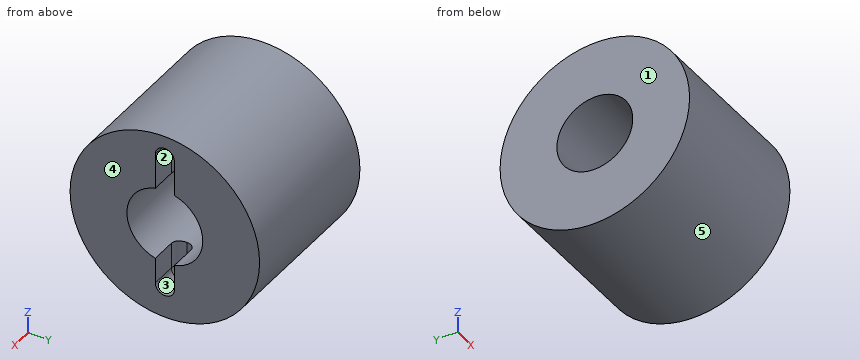
```python
from build123d import *

# Parameters (mm, degrees)
F0_R     = 14.985
F0_R_2   = 6
F1_DEPTH = 25
F3_DEPTH = 5.5
F4_R     = 1.5


with BuildPart() as f1:
    # F0 (on Right) → F1 (new body)
    with BuildSketch(Plane.YZ):
        Circle(F0_R)
        Circle(F0_R_2, mode=Mode.SUBTRACT)
    extrude(amount=-F1_DEPTH)

    # F2 (on Right) → F3 (cut)
    with BuildSketch(Plane.YZ):
        with BuildLine():
            ThreePointArc((1.51, 11.49), (0, 13), (-1.51, 11.49))
            Line((-1.51, 11.49), (-1.51, -9.89))
            ThreePointArc((-1.51, -9.89), (0, -11.4), (1.51, -9.89))
            Line((1.51, -9.89), (1.51, 11.49))
        make_face()
    extrude(amount=-F3_DEPTH, mode=Mode.SUBTRACT)

    # F4
    f4_edges = [f1.edges().sort_by_distance(p)[0] for p in [
        (-5.5, 1.51, 8.648442),
        (-5.5, 1.51, -7.848442),
    ]]
    fillet(f4_edges, radius=F4_R)


solid = f1.part
```
Work out the finished part from the listing and answer in its coordinate system (mm). Face numbers are marked on the shaded views. A direction names the side the tool comes from. Give positions to 0.01 mm unless a question says otherwise; leave off trailing zeros. Write each loop counter-clockwise with the first axis right and the second up, starting at its lowest first coordinate (ties: lowest second). Pieces come first, ordered by that corner, then holes. Notation, with made-up numbers: (-30.75, 30) -> (-1.75, 30) arc R21 cw to (-1.75, 66) -> close; hole circle Ø7 at (-30, 81). An arc over 180 degrees is marked (long way). Write item = value, one per line.
Q1. Consider line 1 along Z through (x, y) = (-18, 0) (3 decimals); line 2 along Y through (x, z) = (-13, 1); line 3 along Y through (x, z) = (-4.25, 11). Determine where each line is inside the solid, lowest interval first.
Computed values:
line_1 = -14.985 to -6, 6 to 14.985
line_2 = -14.95 to -5.92, 5.92 to 14.95
line_3 = -10.18 to -1.49, 1.49 to 10.18
Q2. Flat-ended cylindrical pins translate along their axes: pin 1 Ø1.2 at (x, z) = (-2, 7.5) entering from -Y; pin 2 Ø3 at (x, z) = (-3, -7.5) entering from +Y; pin 3 Ø4 at (x, z) = (-13.5, 3) entering from -Y. Find the tip coordinate at first contact, or state that the pin passes through.
Computed values:
pin_1 = -13.3
pin_2 = 13.73
pin_3 = -14.95
Q3. A tool of negligible diameter and unlimited length cuts with its end or side. For the marked faces 1 and 2, from which of +Z, -Z, +X, -X, +Y, -Y can it reach the whole face along a straight path? Write none if from no direction.
Computed values:
face_1 = +Z, -Z, -X, +Y, -Y
face_2 = +X
Q4. For a pull along Z with two mould halves and no side action, classify the marked faces 3, 4 and 5 as pulls with the +Z half, pulls with the -Z half, needs draft (parallel to the pull), parting line crosses it, or undercut.
Computed values:
face_3 = undercut
face_4 = needs draft
face_5 = parting line crosses it
Q5. Section D-D on y = 11 is taken. Determine the outline of the cut face in (x, z).
Computed values:
outline = (-25, -10.18) -> (0, -10.18) -> (0, 10.18) -> (-25, 10.18) -> close
Q6. Section A-A on z = 0 is taken. Determine the outline of the cut face in (x, y) (3 decimals), and give its area (3 significant figures).
Computed values:
outline = (-25, -14.985) -> (0, -14.985) -> (0, -6) -> (-25, -6) -> close; (-25, 6) -> (0, 6) -> (0, 14.985) -> (-25, 14.985) -> close
area = 449 mm^2
Q7. Section B-B on x = -3 is taken. Determine the outline of the cut face in (y, z) (3 decimals).
Computed values:
outline = circle Ø29.97 at (0, 0); hole (-1.51, -9.89) arc R1.51 ccw to (1.51, -9.89) -> (1.51, -5.807) arc R6 ccw to (1.51, 5.807) -> (1.51, 11.49) arc R1.51 ccw to (-1.51, 11.49) -> (-1.51, 5.807) arc R6 ccw to (-1.51, -5.807) -> close
Q8. Section C-C on y = 4 is taken. Determine the outline of the cut face in (x, z).
Computed values:
outline = (-25, -14.44) -> (0, -14.44) -> (0, -4.47) -> (-25, -4.47) -> close; (-25, 4.47) -> (0, 4.47) -> (0, 14.44) -> (-25, 14.44) -> close
